Autodesk Inventor part; units mm, degrees
ref_plane "YZ Plane" through (0, 0, 0) normal (1, 0, 0) x (0, 1, 0)
ref_plane "XZ Plane" through (0, 0, 0) normal (0, 1, 0) x (-1, 0, 0)
ref_plane "XY Plane" through (0, 0, 0) normal (0, 0, 1) x (1, 0, 0)
sketch "Sketch1" plane through (0, 0, 0) normal (0, 0, 1) x (1, 0, 0)
  circle A0 centre (0, 0) radius 7.5
  dimension "d0" = 15
extrude "Extrusion1" add sketch "Sketch1" against normal blind 6
sketch "Sketch2" plane through (0, 0, -6) normal (0, 0, -1) x (-1, 0, 0)
  circle A0 centre (0, 0) radius 6
  dimension "d3" = 12
extrude "Extrusion2" add sketch "Sketch2" along normal blind 5
sketch "Sketch3" plane through (0, 0, -11) normal (0, 0, -1) x (-1, 0, 0)
  circle A0 centre (0, 0) radius 6
hole "Hole1" at (0, 0, -11) direction (0, 0, 1) diameter 8 depth 11
thread "Thread1"
properties part number "117" material "Aluminum 6061"
Here's how the part is built. I have some questions about the finished solid (model axes, mm). Coordinates: 2 decimals unless noted, no trailing zeros. Write each loop counter-clockwise with the first axis right and the second up, starting at its lowest first coordinate (ties: lowest second). Pieces come first, ordered by that corner, then holes.
1) If I drill on line 1 (Y direction, x = 0, z = -8); line 2 (Y direction, x = 0, z = -4); line 3 (X direction, y = -3, z = -10), over which ranges is the centre line in solid material (lowest first)?
Filled in:
line 1: y = -6 to -4, 4 to 6
line 2: y = -7.5 to -4, 4 to 7.5
line 3: x = -5.2 to -2.65, 2.65 to 5.2
2) Thinking about a two-plate mould opening in X: for faces 1 (the face through (2, 6, -6)), 2 (the face through (6, 0, -8)), 3 (the face through (3.905, -0.867, -5.423)), which applies, +X half, -X half, draft (parallel to the pull), parting line (faces both ways), or undercut?
Filled in:
face 1: draft
face 2: parting line
face 3: undercut
3) If we section it at C-C (z = -3.75): List the corners of the cut face in (x, y) for me, plus the area to 3 significant figures.
Filled in:
outline: circle Ø15 at (0, 0); hole circle Ø8 at (0, 0)
area: 126 mm2
4) I'm going to push flat-ended pins straight in: pin 1 (1.5 mm diameter, centred on x = 5, y = -6, fed in from -Z); pin 2 (5 mm diameter, centred on y = -5, z = -6, fed in from +X); pin 3 (6 mm diameter, centred on y = -4, z = -9.5, fed in from +X). Where does each tip first touch, or does it pass through?
Filled in:
pin 1: stops at z = -6
pin 2: stops at x = 7.07
pin 3: stops at x = 5.92
5) If we section it at D-D (y = 5.5): List the corners of the cut face in (x, z) for me, plus the area to 3 significant figures.
Filled in:
outline: (-5.1, -6) - (-2.4, -6) - (-2.4, -11) - (2.4, -11) - (2.4, -6) - (5.1, -6) - (5.1, 0) - (-5.1, 0) - close
area: 85.2 mm2
6) If we section it at A-A (y = 0): List the corners of the cut face in (x, z) for me.
Filled in:
outline: (-7.5, -6) - (-6, -6) - (-6, -11) - (-4, -11) - (-4, 0) - (-7.5, 0) - close; (4, -11) - (6, -11) - (6, -6) - (7.5, -6) - (7.5, 0) - (4, 0) - close
